Source: CAD feature listing. Evaluate the final solid. Frame: model axes, mm. Face numbers are marked on the shaded views. A direction names the side the tool comes from. Give positions to 0.01 mm unless a question says otherwise; leave off trailing zeros. Order: outer loops, then holes, each group sorted by start corner. A loop starts at its lowest first (then second) coordinate and runs counter-clockwise, first axis right, second up.
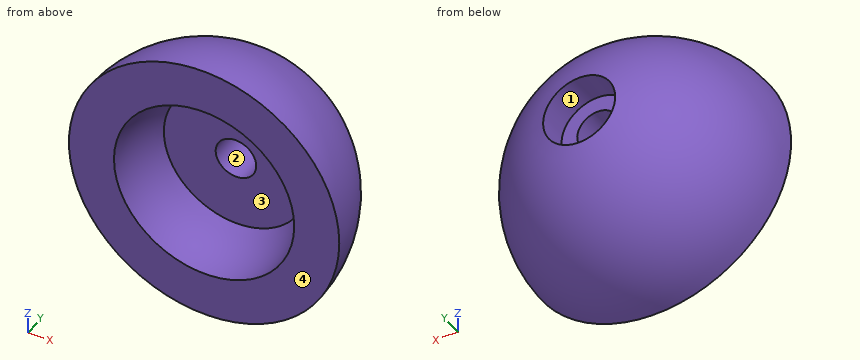
Autodesk Inventor part; units mm, degrees
ref_plane "Work Plane1" through (0, 15, 0) normal (0, 1, 0) x (-1, 0, 0)
ref_plane "YZ Plane" through (0, 0, 0) normal (1, 0, 0) x (0, 1, 0)
ref_plane "XY Plane" through (0, 0, 0) normal (0, 0, 1) x (1, 0, 0)
sketch "Sketch1" plane through (0, 0, 0) normal (0, 0, 1) x (1, 0, 0)
  line L0 (0, 0) -> (0, 15)
  line L1 (0, 0) -> (15, 0)
  arc A0 (15, 0) -> (0, 15) centre (0, 0) ccw
  line L2 (0, -3.6213) -> (0, 21.7279)
  dimension "d2" = 15
revolve "Revolution1" add sketch "Sketch1" angle 360 about axis through (0, -10, 0) along (0, 1, 0)
ref_plane "Work Plane1" through (0, 15, 0) normal (0, 1, 0) x (-1, 0, 0)
sketch "Sketch2" plane through (0, 15, 0) normal (0, 1, 0) x (-1, 0, 0)
  point P0 (0, 0)
  point P1 (0, 0)
hole "Hole1" at (0, 15, 0) direction (0, -1, 0) diameter 4.5 end through all counterbore diameter 8 counterbore depth 4
shell "Shell1" thickness 5 removed faces 1 at (10.5992, 0, 1.287)
sketch "Sketch3" plane through (0, 0, 0) normal (0, -1, 0) x (1, 0, 0)
  circle A0 centre (0, 0) radius 7.25
  circle A1 centre (0, 0) radius 2.25
extrude "Extrusion1" cut sketch "Sketch3" against normal blind 6
properties part number "Ball_Upper Half" material "Nylon 6/6"
1) Pin query (flat end, axial travel): pin 1 (6 mm diameter, centred on y = 9.5, z = -5, fed in from -X); pin 2 (5 mm diameter, centred on x = -1, y = 12.5, fed in from +Z); pin 3 (5 mm diameter, centred on x = 0, z = 0, fed in from -Y). Return the tip coordinate at first contact, or that it passes through.
Report:
pin 1: stops at x = -12.85
pin 2: stops at z = 11.14
pin 3: stops at y = 6
2) Reachability of the marked faces 1 and 2 from +Z, -Z, +X, -X, +Y, -Y: full face, straight path, thin tool, end or side. Return the list, or none.
Report:
face 1: +Y
face 2: +Y, -Y
3) Section query B-B, the plane y = 12. Return the cut outline in (x, z), and give its area (3 significant figures).
Report:
outline: circle Ø18 at (0, 0); hole circle Ø8 at (0, 0)
area: 204 mm2
4) Section query C-C, the plane z = 12. Return the cut outline in (x, y), and give its area (3 significant figures).
Report:
outline: (-9, 0) - (9, 0) arc R9 ccw to start
area: 127 mm2
5) Section query A-A, the plane z = 0. Return the cut outline in (x, y), and give its area (3 significant figures).
Report:
outline: (-15, 0) - (-10, 0) arc R10 cw to (-8, 6) - (-2.25, 6) - (-2.25, 11) - (-4, 11) - (-4, 14.46) arc R15 ccw to start; (2.25, 6) - (8, 6) arc R10 cw to (10, 0) - (15, 0) arc R15 ccw to (4, 14.46) - (4, 11) - (2.25, 11) - close
area: 188 mm2
6) Section query D-D, the plane x = 12.25. Return the cut outline in (y, z), and give its area (3 significant figures).
Report:
outline: (0, -8.66) arc R8.66 ccw to (0, 8.66) - close
area: 118 mm2
7) Draft query along X for the marked faces 3 and 4. Return one class per face: +X half, -X half, draft (parallel to the pull), parting line (faces both ways), or undercut.
Report:
face 3: undercut
face 4: draft
8) Material intervals for L1, parallel to X at y = 10, z = 0; L2, parallel to Y at x = 2.5, z = -3; L3, parallel to X at y = 12.7, z = 0, sorted ascending.
Report:
L1: x = -11.18 to -2.25, 2.25 to 11.18
L2: y = 6 to 11
L3: x = -7.98 to -4, 4 to 7.98
